For this review, take the finished solid that the model builds, in its own axes (mm). Face numbers are marked on the shaded views. Give positions to 0.01 mm unless a question says otherwise; leave off trailing zeros. Loops run counter-clockwise (first coordinate to the right, second up) from the corner with the lowest first, then second, coordinate; pieces in that order, holes last.
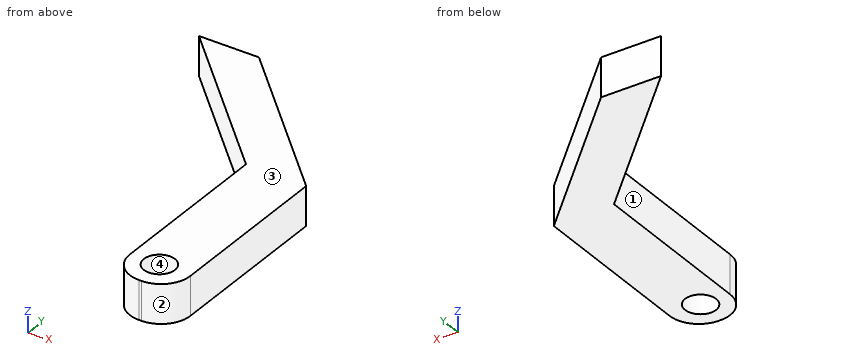
Autodesk Inventor part; units mm, degrees
ref_plane "YZ Plane" through (0, 0, 0) normal (1, 0, 0) x (0, 1, 0)
ref_plane "XZ Plane" through (0, 0, 0) normal (0, 1, 0) x (-1, 0, 0)
ref_plane "XY Plane" through (0, 0, 0) normal (0, 0, 1) x (1, 0, 0)
sketch "Szkic1" plane through (0, 0, 0) normal (0, 0, 1) x (1, 0, 0)
  circle A0 centre (3, 5) radius 1.45
  circle A1 centre (3, 5) radius 1.6
  line L0 (6.229, 0) -> (6.229, 8)
  line L1 (0, 0) -> (0, 8)
  line L2 (3.229, 1.9318) -> (3, 1.9318)
  line L3 (0, 4.9318) -> (0, 22.5946)
  line L4 (6.229, 22.5402) -> (6.229, 4.9318)
  arc A2 (3.229, 1.9318) -> (6.229, 4.9318) centre (3.229, 4.9318) ccw
  arc A3 (0, 4.9318) -> (3, 1.9318) centre (3, 4.9318) ccw
  line L5 (0, 22.5946) -> (-14.9838, 37.5785)
  line L6 (6.229, 22.5402) -> (-8.8092, 37.5785)
  line L7 (-8.8092, 37.5785) -> (-14.9838, 37.5785)
  point P0 (6.229, 1.9318)
  dimension "d0" = 3.2
  dimension "d1" = 3
  dimension "d2" = 135
extrude "Wyciągnięcie proste1" add sketch "Szkic1" along normal blind 4 contours A2 L2 A3 L1 L3 L5 L7 L6 L4 L0
properties part number "mirror_holder"
Q1. Consider section A-A on z = 1.9. Give the boundary of the cut face in (x, y), plus the area to 3 significant figures.
Answers:
outline: (-14.98, 37.58) - (0, 22.59) - (0, 4.93) arc R3 ccw to (3, 1.93) - (3.23, 1.93) arc R3 ccw to (6.23, 4.93) - (6.23, 22.54) - (-8.81, 37.58) - close; hole circle Ø3.2 at (3, 5)
area: 209 mm2
Q2. For probe 1 along X at (y, z) = (8.5, 3.5); probe 2 along X at (y, z) = (4.5, 2.45); probe 3 along Y at (x, z) = (3, 1.85), list the stretches that pass through material, from the lowest coordinate up.
Answers:
probe 1: x = 0 to 6.23
probe 2: x = 0.03 to 1.48, 4.52 to 6.2
probe 3: y = 1.93 to 3.4, 6.6 to 25.77
Q3. Consider section C-C on x = -11. Give the boundary of the cut face in (y, z), plus the area to 3 significant figures.
Answers:
outline: (33.59, 0) - (37.58, 0) - (37.58, 4) - (33.59, 4) - close
area: 15.9 mm2
Q4. Consider section B-B on y = 7.5. Give the boundary of the cut face in (x, z), plus the area to 3 significant figures.
Answers:
outline: (0, 0) - (6.23, 0) - (6.23, 4) - (0, 4) - close
area: 24.9 mm2
Q5. Mouldability with a two-part tool opening along X and no side actions: class the marked faces 1, 2, 3 and 4 as +X half, -X half, draft (parallel to the pull), parting line (faces both ways), or undercut.
Answers:
face 1: -X half
face 2: +X half
face 3: draft
face 4: undercut
Q6. For pin 1 Ø1 at (x, z) = (-4.5, 1.5) entering from +Y; pin 2 Ø1.2 at (y, z) = (18, 2) entering from -X, all flat-tipped, find the tip position at first contact; note any pin that passes through.
Answers:
pin 1: stops at y = 33.77
pin 2: stops at x = 0
